```python
from build123d import *

# Parameters (mm, degrees)
SKETCH_1_W          = 100
SKETCH_1_H          = 80
EXTRUDE_1_DEPTH     = 4
SKETCH_2_W          = 5
SKETCH_2_H          = 80
EXTRUDE_2_DEPTH     = 50
CUT_EXTRUDE_2_DEPTH = 5
FILLET_1_R          = 10
FILLET_2_R          = 3
FILLET_3_R          = 3
SKETCH_5_R          = 2.1
CUT_EXTRUDE_3_DEPTH = 5
SKETCH_6_R          = 2.5
CUT_EXTRUDE_4_DEPTH = 10
SKETCH_7_W          = 22
SKETCH_7_H          = 42
CUT_EXTRUDE_5_DEPTH = 10
SKETCH_8_W          = 22
SKETCH_8_H          = 42
CUT_EXTRUDE_6_DEPTH = 10
FILLET_4_R          = 0.5
FILLET_5_R          = 0.5
SKETCH_9_W          = 5
SKETCH_9_H          = 27
EXTRUDE_3_DEPTH     = 40
CUT_EXTRUDE_7_DEPTH = 20
SKETCH_11_W         = 5
SKETCH_11_H         = 20
EXTRUDE_4_DEPTH     = 20
FILLET_6_RADIUS     = 10
FILLET_6_LENGTH     = 5
FILLET_7_R          = 3
SKETCH_12_R         = 2.1
CUT_EXTRUDE_8_DEPTH = 20


with BuildPart() as part:
    # 草图1 → 凸台-拉伸1 (new body)
    with BuildSketch(Plane.XY):
        with Locations((50, 40)):
            Rectangle(SKETCH_1_W, SKETCH_1_H)
    extrude(amount=EXTRUDE_1_DEPTH)

    # 草图2 → 凸台-拉伸2 (add)
    with BuildSketch(Plane.XY.offset(4)):
        with Locations((2.5, 40)):
            Rectangle(SKETCH_2_W, SKETCH_2_H)
        with Locations((97.5, 40)):
            Rectangle(SKETCH_2_W, SKETCH_2_H)
        with Locations((50, 40)):
            Rectangle(SKETCH_2_W, SKETCH_2_H)
    extrude(amount=EXTRUDE_2_DEPTH)

    # 草图4 → 切除-拉伸2 (cut)
    with BuildSketch(Plane.ZY.offset(-47.5)):
        Polygon((54, 80), (4, 80), (54, 40), align=None)
        Polygon((54, 0), (54, 40), (4, 0), align=None)
    extrude(amount=-CUT_EXTRUDE_2_DEPTH, mode=Mode.SUBTRACT)

    # 圆角1
    fillet_1_edges = [part.edges().sort_by_distance(p)[0] for p in [
        (50, 40, 54),
    ]]
    fillet(fillet_1_edges, radius=FILLET_1_R)

    # 圆角2
    fillet_2_edges = [part.edges().sort_by_distance(p)[0] for p in [
        (5, 40, 4),
        (2.5, 0, 54),
        (2.5, 80, 54),
        (95, 40, 4),
        (97.5, 80, 54),
        (97.5, 0, 54),
    ]]
    fillet(fillet_2_edges, radius=FILLET_2_R)

    # 圆角3
    fillet_3_edges = [part.edges().sort_by_distance(p)[0] for p in [
        (47.5, 40, 4),
        (52.5, 40, 4),
    ]]
    fillet(fillet_3_edges, radius=FILLET_3_R)

    # 草图5 → 切除-拉伸3 (cut)
    with BuildSketch(Plane(origin=(0, 0, 0), x_dir=(-1, 0, 0), z_dir=(0, 0, -1))):
        with Locations((-65, 50)):
            Circle(SKETCH_5_R)
        with Locations((-35, 50)):
            Circle(SKETCH_5_R)
        with Locations((-65, 30)):
            Circle(SKETCH_5_R)
        with Locations((-35, 30)):
            Circle(SKETCH_5_R)
    extrude(amount=-CUT_EXTRUDE_3_DEPTH, mode=Mode.SUBTRACT)

    # 草图6 → 切除-拉伸4 (cut)
    with BuildSketch(Plane.ZY.offset(-47.5)):
        with Locations(Location((37.992189406, 40, 0), (0, 0, 270))):
            Circle(SKETCH_6_R)
    extrude(amount=-CUT_EXTRUDE_4_DEPTH, mode=Mode.SUBTRACT)

    # 草图7 → 切除-拉伸5 (cut)
    with BuildSketch(Plane.ZY):
        with Locations((38, 30)):
            Rectangle(SKETCH_7_W, SKETCH_7_H)
    extrude(amount=-CUT_EXTRUDE_5_DEPTH, mode=Mode.SUBTRACT)

    # 草图8 → 切除-拉伸6 (cut)
    with BuildSketch(Plane(origin=(100, 0, 0), x_dir=(0, 0, -1), z_dir=(1, 0, 0))):
        with Locations((-38, 30)):
            Rectangle(SKETCH_8_W, SKETCH_8_H)
    extrude(amount=-CUT_EXTRUDE_6_DEPTH, mode=Mode.SUBTRACT)

    # 圆角4
    fillet_4_edges = [part.edges().sort_by_distance(p)[0] for p in [
        (97.5, 9, 49),
        (97.5, 51, 49),
        (97.5, 51, 27),
        (97.5, 9, 27),
    ]]
    fillet(fillet_4_edges, radius=FILLET_4_R)

    # 圆角5
    fillet_5_edges = [part.edges().sort_by_distance(p)[0] for p in [
        (2.5, 9, 27),
        (2.5, 51, 27),
        (2.5, 51, 49),
        (2.5, 9, 49),
    ]]
    fillet(fillet_5_edges, radius=FILLET_5_R)

    # 草图9 → 凸台-拉伸3 (add)
    with BuildSketch(Plane(origin=(0, 80, 0), x_dir=(1, 0, 0), z_dir=(0, 1, 0))):
        with Locations((2.5, -30.5)):
            Rectangle(SKETCH_9_W, SKETCH_9_H)
    extrude(amount=EXTRUDE_3_DEPTH)

    # 草图10 → 切除-拉伸7 (cut)
    with BuildSketch(Plane.ZY):
        Polygon((17, 80), (30.5, 120), (17, 120), align=None)
    extrude(amount=-CUT_EXTRUDE_7_DEPTH, mode=Mode.SUBTRACT)

    # 草图11 → 凸台-拉伸4 (add)
    with BuildSketch(Plane.XY.offset(44)):
        with Locations((2.5, 110)):
            Rectangle(SKETCH_11_W, SKETCH_11_H)
    extrude(amount=EXTRUDE_4_DEPTH)

    # 圆角6: full round fillet: the end face becomes a half cylinder, R = half its width
    fillet_6_face = Plane((2.5, 110, 64), x_dir=(1, 0, 0), z_dir=(0, 0, 1))  # on the end face: x along it, z out of the body
    fillet_6_slab = fillet_6_face.offset(-FILLET_6_RADIUS / 2) * Box(FILLET_6_LENGTH, 2 * FILLET_6_RADIUS, FILLET_6_RADIUS, mode=Mode.PRIVATE)  # the body's end, R deep
    fillet_6_round = Plane((2.5, 110, 54), x_dir=(0, 0, 1), z_dir=(1, 0, 0)) * Cylinder(FILLET_6_RADIUS, FILLET_6_LENGTH, mode=Mode.PRIVATE)  # its axis R under the face
    add(fillet_6_slab - fillet_6_round, mode=Mode.SUBTRACT)

    # 圆角7
    fillet_7_edges = [part.edges().sort_by_distance(p)[0] for p in [
        (2.5, 80, 44),
        (2.5, 80, 17),
        (2.5, 120, 30.5),
        (2.5, 100, 44),
    ]]
    fillet(fillet_7_edges, radius=FILLET_7_R)

    # 草图12 → 切除-拉伸8 (cut)
    with BuildSketch(Plane.ZY):
        with Locations((54, 110)):
            Circle(SKETCH_12_R)
    extrude(amount=-CUT_EXTRUDE_8_DEPTH, mode=Mode.SUBTRACT)


solid = part.part
```
Source: CAD feature listing. Evaluate the final solid. Frame: model axes, mm. A direction names the side the tool comes from. Coordinates: 2 decimals unless noted, no trailing zeros. Write each loop counter-clockwise with the first axis right and the second up, starting at its lowest first coordinate (ties: lowest second). Pieces come first, ordered by that corner, then holes. Notation, with made-up numbers: (66, 82.25) -> (107, 82.25) arc R19 ccw to (107, 97.25) -> close; hole circle Ø9 at (66, 81.25). An arc over 180 degrees is marked (long way). Return JSON: item names as keys, results as strings. Group by question number.
1) Set-up query: faces 1 (the face through (5, 59, 29)), 2 (the face through (98, 9, 38)), 3 (the face through (2, 30, 27)), 4 (the face through (2, 90, 44)), 5 (the face through (2.54, 119.42, 30.88)). Return all of +Z, -Z, +X, -X, +Y, -Y with unobstructed straight access to the full face (end or side cutting, diameter ignored); none if empty.
2) Section query A-A, the plane x = 35. Return loops of the section in (y, z), plus the area to 3 significant figures.
3) Contact query for flat-ended pins moving along their axis: P1, Ø4, axis at y = 87.5, z = 27, coming from the +X side; P2, Ø1.5, axis at x = 2, y = 91.5, coming from the +Z side; P3, Ø2.5, axis at x = 98.5, y = 31, coming from the +Z side; P4, Ø2, axis at y = 16, z = 13, coming from the -X side. Output: stop coordinate, or through.
4) Mould query, pull axis Z, two halves, no side actions, for faces 6 (the face through (2.535, 80.548, 16.575)), 7 (the face through (61, 80, 3)), 8 (the face through (50, 64, 24)), 9 (the face through (98, 30, 27)). Classes: +Z half, -Z half, draft (parallel to the pull), parting line (faces both ways), or undercut.
5) Section query B-B, the plane y = 17. Return loops of the section in (x, z), plus the area to 3 significant figures.
6) Section query C-C, the plane y = 30. State how many separate pieces and enclosed holes the cut face has, plus the area to 3 significant figures.
7) Section query D-D, the plane y = 110. Return loops of the section in (x, z) (3 decimals).
8) Ray query, line 1 along Y through (x, z) = (35, 2.9); line 2 along X through (y, z) = (54, 28.5); line 3 along X through (y, z) = (78.5, 43). Return the intervals inside material, ascending.
From the geometry:
{
 "1": {"face 1": "+Z, +Y, -Y", "face 2": "+X, -X", "face 3": "-X", "face 4": "+Z, +X, -X", "face 5": "-Z, +X, -X, +Y"},
 "2": {"outline": "(0, 0) -> (27.9, 0) -> (27.9, 4) -> (0, 4) -> close; (32.1, 0) -> (47.9, 0) -> (47.9, 4) -> (32.1, 4) -> close; (52.1, 0) -> (80, 0) -> (80, 4) -> (52.1, 4) -> close", "area": "286 mm²"},
 "3": {"P1": "x = 5", "P2": "z = 44", "P3": "z = 54", "P4": "x = 0"},
 "4": {"face 6": "-Z half", "face 7": "draft", "face 8": "+Z half", "face 9": "undercut"},
 "5": {"outline": "(0, 0) -> (100, 0) -> (100, 27) -> (95, 27) -> (95, 7) arc R3 cw to (92, 4) -> (55.5, 4) arc R3 cw to (52.5, 7) -> (52.5, 25.25) -> (47.5, 25.25) -> (47.5, 7) arc R3 cw to (44.5, 4) -> (8, 4) arc R3 cw to (5, 7) -> (5, 27) -> (0, 27) -> close; (0, 49) -> (5, 49) -> (5, 54) -> (0, 54) -> close; (95, 49) -> (100, 49) -> (100, 54) -> (95, 54) -> close", "area": "794 mm²"},
 "6": {"separate pieces": "5", "enclosed holes": "0", "area": "842 mm²"},
 "7": {"outline": "(0, 27.125) -> (5, 27.125) -> (5, 51.9) -> (0, 51.9) -> close; (0, 56.1) -> (5, 56.1) -> (5, 64) -> (0, 64) -> close"},
 "8": {"line 1": "0 to 27.9, 32.1 to 47.9, 52.1 to 80", "line 2": "0 to 5, 47.5 to 52.5, 95 to 100", "line 3": "0 to 5, 95 to 100"}
}
